Input: part model. Units: mm. Frame: model coordinates. Face numbers are marked on the shaded views. A direction names the side the tool comes from. Give positions to 0.01 mm unless a question says otherwise; leave off trailing zeros. Loops run counter-clockwise (first coordinate to the right, second up) from the corner with the lowest first, then second, coordinate; pieces in that order, holes last. Notation, with made-up numbers: (-17.5, -18) -> (-3.5, -18) arc R17 cw to (-3.5, 9) -> close; hole circle Ø7 at (10, 24.5). An arc over 180 degrees is marked (long way). Answer in a Markdown table with one row per item. Add a question column.
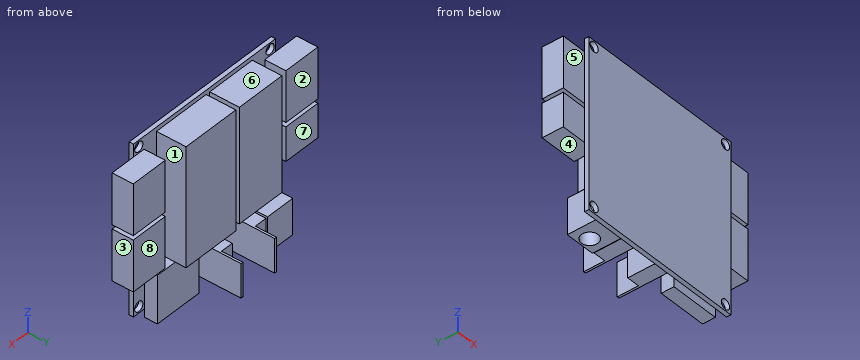
```python
from build123d import *

# Parameters (mm, degrees)
SKETCH5_W           = 50.8
SKETCH5_H           = 50.8
BOSS_EXTRUDE1_DEPTH = 1.27
SKETCH6_W           = 11.43
SKETCH6_H           = 10.16
SKETCH6_H_2         = 15.24
BOSS_EXTRUDE2_DEPTH = 6.35
SKETCH7_W           = 15.24
SKETCH7_H           = 34.29
SKETCH7_W_2         = 17.78
SKETCH7_H_2         = 35.56
BOSS_EXTRUDE3_DEPTH = 8.89
SKETCH8_R           = 1.4732
CUT_EXTRUDE1_DEPTH  = 2.27
SKETCH9_W           = 4.445
SKETCH9_H           = 10.16
BOSS_EXTRUDE4_DEPTH = 8.89
SKETCH11_W          = 0.635
SKETCH11_H          = 10.16
BOSS_EXTRUDE5_DEPTH = 6.35
SKETCH12_W          = 8.999982
SKETCH12_H          = 10.700004
BOSS_EXTRUDE6_DEPTH = 8.89
SKETCH13_W          = 14.8000212
SKETCH13_H          = 14.2999968
BOSS_EXTRUDE7_DEPTH = 3.81
SKETCH17_R          = 2.5
CUT_EXTRUDE2_DEPTH  = 6.35


with BuildPart() as part:
    # Sketch5 → Boss-Extrude1 (new body)
    with BuildSketch(Plane(origin=(0, 0, 0), x_dir=(1, 0, 0), z_dir=(0, 1, 0))):
        with Locations((25.4, 25.4)):
            Rectangle(SKETCH5_W, SKETCH5_H)
    extrude(amount=-BOSS_EXTRUDE1_DEPTH)

    # Sketch6 → Boss-Extrude2 (add)
    with BuildSketch(Plane(origin=(0, 0, 0), x_dir=(1, 0, 0), z_dir=(0, 1, 0))):
        with Locations((-1.905, 25.4)):
            Rectangle(SKETCH6_W, SKETCH6_H)
        with Locations((-1.905, 11.43)):
            Rectangle(SKETCH6_W, SKETCH6_H_2)
        with Locations((52.705, 27.94)):
            Rectangle(SKETCH6_W, SKETCH6_H_2)
        with Locations((52.705, 11.43)):
            Rectangle(SKETCH6_W, SKETCH6_H_2)
    extrude(amount=BOSS_EXTRUDE2_DEPTH)

    # Sketch7 → Boss-Extrude3 (add)
    with BuildSketch(Plane(origin=(0, 0, 0), x_dir=(1, 0, 0), z_dir=(0, 1, 0))):
        with Locations((15.875, 18.415)):
            Rectangle(SKETCH7_W, SKETCH7_H)
        with Locations((33.655, 19.05)):
            Rectangle(SKETCH7_W_2, SKETCH7_H_2)
    extrude(amount=BOSS_EXTRUDE3_DEPTH)

    # Sketch8 → Cut-Extrude1 (cut, through all)
    with BuildSketch(Plane(origin=(0, 0, 0), x_dir=(1, 0, 0), z_dir=(0, 1, 0))):
        with Locations((1.905, 48.895)):
            Circle(SKETCH8_R)
        with Locations((48.895, 48.895)):
            Circle(SKETCH8_R)
        with Locations((1.905, 1.905)):
            Circle(SKETCH8_R)
        with Locations((48.895, 1.905)):
            Circle(SKETCH8_R)
    extrude(amount=-CUT_EXTRUDE1_DEPTH, mode=Mode.SUBTRACT)

    # Sketch9 → Boss-Extrude4 (add)
    with BuildSketch(Plane(origin=(0, 0, 0), x_dir=(1, 0, 0), z_dir=(0, 1, 0))):
        with Locations((28.2575, 44.7675)):
            Rectangle(SKETCH9_W, SKETCH9_H)
        with Locations((16.1925, 44.7675)):
            Rectangle(SKETCH9_W, SKETCH9_H)
    extrude(amount=BOSS_EXTRUDE4_DEPTH)

    # Sketch11 → Boss-Extrude5 (add)
    with BuildSketch(Plane(origin=(0, 8.89, 0), x_dir=(1, 0, 0), z_dir=(0, 1, 0))):
        with Locations((30.1625, 44.7675)):
            Rectangle(SKETCH11_W, SKETCH11_H)
        with Locations((18.0975, 44.7675)):
            Rectangle(SKETCH11_W, SKETCH11_H)
    extrude(amount=BOSS_EXTRUDE5_DEPTH)

    # Sketch12 → Boss-Extrude6 (add)
    with BuildSketch(Plane(origin=(0, 0, 0), x_dir=(1, 0, 0), z_dir=(0, 1, 0))):
        with Locations((8.89, 44.990004)):
            Rectangle(SKETCH12_W, SKETCH12_H)
    extrude(amount=BOSS_EXTRUDE6_DEPTH)

    # Sketch13 → Boss-Extrude7 (add)
    with BuildSketch(Plane(origin=(0, 0, 0), x_dir=(1, 0, 0), z_dir=(0, 1, 0))):
        with Locations((39.37, 46.219999)):
            Rectangle(SKETCH13_W, SKETCH13_H)
    extrude(amount=BOSS_EXTRUDE7_DEPTH)

    # Sketch17 → Cut-Extrude2 (cut)
    with BuildSketch(Plane(origin=(0, 0, -50.340006), x_dir=(-1, 0, 0), z_dir=(0, 0, -1))):
        with Locations((-8.89, 5.916248933)):
            Circle(SKETCH17_R)
    extrude(amount=-CUT_EXTRUDE2_DEPTH, mode=Mode.SUBTRACT)


solid = part.part
```
1) Pull-direction query (X, two-part tool) for the marked faces 1, 2 and 3; classes: +X half, -X half, draft (parallel to the pull), parting line (faces both ways), or undercut.
2) Material intervals for line 1 along X through (y, z) = (5.5, -42) (3 decimals); line 2 along X through (y, z) = (5.75, -30) (3 decimals); line 3 along Z through (x, y) = (17.5, 8), sorted ascending.
3) Section D-D on z = -23.5. Output: boundary loops of the cut face in (x, y) (3 decimals).
4) Pin query (flat end, axial travel): pin 1 (6 mm diameter, centred on x = 29.5, z = -8.5, fed in from +Y); pin 2 (3 mm diameter, centred on x = 44.5, z = -13, fed in from +Y); pin 3 (11 mm diameter, centred on x = -2, z = -25.5, fed in from +Y). Return the tip coordinate at first contact, or that it passes through.
5) Section C-C on x = 15. Output: boundary loops of the cut face in (y, z).
6) Reachability of the marked faces 4, 5, 6, 7 and 8 from +Z, -Z, +X, -X, +Y, -Y: full face, straight path, thin tool, end or side. Return the list, or none.
7) Section A-A on y = 10.25. Output: boundary loops of the cut face in (x, z) (1 decimal), and give its area (3 significant figures).
8) Section B-B on z = -32. Output: boundary loops of the cut face in (x, y) (3 decimals), and give its area (3 significant figures).
Working result:
| question | item | result |
|---|---|---|
| 1 | face 1 | undercut |
| 1 | face 2 | draft |
| 1 | face 3 | +X half |
| 2 | line 1 | x = 4.39 to 13.39, 13.97 to 18.415, 26.035 to 30.48 |
| 2 | line 2 | x = -7.62 to 3.81, 8.255 to 23.495, 24.765 to 42.545, 46.99 to 58.42 |
| 2 | line 3 | z = -49.85 to -39.69, -35.56 to -1.27 |
| 3 | outline | (-7.62, 0) -> (0, 0) -> (0, -1.27) -> (50.8, -1.27) -> (50.8, 0) -> (58.42, 0) -> (58.42, 6.35) -> (46.99, 6.35) -> (46.99, 0) -> (42.545, 0) -> (42.545, 8.89) -> (24.765, 8.89) -> (24.765, 0) -> (23.495, 0) -> (23.495, 8.89) -> (8.255, 8.89) -> (8.255, 0) -> (3.81, 0) -> (3.81, 6.35) -> (-7.62, 6.35) -> close |
| 4 | pin 1 | stops at y = 8.89 |
| 4 | pin 2 | stops at y = 0 |
| 4 | pin 3 | stops at y = 6.35 |
| 5 | outline | (-1.27, -50.8) -> (0, -50.8) -> (0, -49.85) -> (8.89, -49.85) -> (8.89, -39.69) -> (0, -39.69) -> (0, -35.56) -> (8.89, -35.56) -> (8.89, -1.27) -> (0, -1.27) -> (0, 0) -> (-1.27, 0) -> close |
| 6 | face 4 | -Z, -X, +Y |
| 6 | face 5 | +Z, -Z, -X, -Y |
| 6 | face 6 | +Z, +X, -X, +Y |
| 6 | face 7 | +Z, -Z, -X, +Y |
| 6 | face 8 | +Z, -Z, +X, +Y |
| 7 | outline | (17.8, -49.8) -> (18.4, -49.8) -> (18.4, -39.7) -> (17.8, -39.7) -> close; (29.8, -49.8) -> (30.5, -49.8) -> (30.5, -39.7) -> (29.8, -39.7) -> close |
| 7 | area | 12.9 mm2 |
| 8 | outline | (0, -1.27) -> (50.8, -1.27) -> (50.8, 0) -> (58.42, 0) -> (58.42, 6.35) -> (46.99, 6.35) -> (46.99, 0) -> (42.545, 0) -> (42.545, 8.89) -> (24.765, 8.89) -> (24.765, 0) -> (23.495, 0) -> (23.495, 8.89) -> (8.255, 8.89) -> (8.255, 0) -> (0, 0) -> close |
| 8 | area | 431 mm2 |
